Source: CAD feature listing. Evaluate the final solid. Frame: model axes, mm. Face numbers are marked on the shaded views. Coordinates: 2 decimals unless noted, no trailing zeros. Write each loop counter-clockwise with the first axis right and the second up, starting at its lowest first coordinate (ties: lowest second). Pieces come first, ordered by that corner, then holes. Notation, with made-up numbers: M 40.25,72.25 L 80.25,72.25 A31 ccw 80.25,98.25 Z; hole C 52.5,-34.75 d2. An arc over 180 degrees is marked long. Answer as CSV lines item,"result". Start each with the question number.
1. Contact query for a flat-ended pin moving along its axis: pin 1 Ø1 at (y, z) = (5, -1.5) entering from +X. Output: stop coordinate, or through.
2. Section A-A on z = 0. Return the cut outline in (x, y), plus the area to 3 significant figures.
3. Line query: probe 1 along X at (y, z) = (4.25, 0); probe 2 along X at (y, z) = (11, -0.55); probe 3 along Z at (x, y) = (0.7, 11). Output: solid intervals per line, ascending. Write a range as [from, to].
4. Mould query, pull axis Z, two halves, no side actions, for the marked faces 1, 2, 3 and 4. Classes: pulls with the +Z half, pulls with the -Z half, needs draft (parallel to the pull), parting line crosses it, or undercut.
5. Section C-C on x = -0.7. Return the cut outline in (y, z).
6. Section D-D on z = -1.5. Return the cut outline in (x, y), plus the area to 3 significant figures.
Autodesk Inventor part; units mm, degrees
ref_plane "YZ Plane" through (0, 0, 0) normal (1, 0, 0) x (0, 1, 0)
ref_plane "XZ Plane" through (0, 0, 0) normal (0, 1, 0) x (-1, 0, 0)
ref_plane "XY Plane" through (0, 0, 0) normal (0, 0, 1) x (1, 0, 0)
sketch "Sketch1" plane through (0, 0, 0) normal (0, 1, 0) x (-1, 0, 0)
  line L0 (1.5155, -0.875) -> (0, -1.75)
  line L1 (0, -1.75) -> (-1.5155, -0.875)
  line L2 (-1.5155, -0.875) -> (-1.5155, 0.875)
  line L3 (-1.5155, 0.875) -> (0, 1.75)
  line L4 (0, 1.75) -> (1.5155, 0.875)
  line L5 (1.5155, 0.875) -> (1.5155, -0.875)
  point P0 (0, 0)
  point P1 (0, 0)
  dimension "d0" = 1.75
extrude "Extrusion1" add sketch "Sketch1" along normal blind 12
sketch "Sketch2" plane through (0, 12, 0) normal (0, 1, 0) x (1, 0, 0)
  point P0 (0, 0)
  point P1 (0, 0)
hole "Hole1" at (0, 12, 0) direction (0, -1, 0) diameter 2.013 end through all
sketch "Sketch3" plane through (0, 0, 0) normal (0, -1, 0) x (1, 0, 0)
  point P0 (-34.949, 34.34)
  point P1 (0, 0)
  point P2 (-40.6419, -41.3626)
  point P3 (-75.5909, -7.0226)
sketch "Sketch4" plane through (0, 12, 0) normal (0, 1, 0) x (1, 0, 0)
  point P0 (0, 0)
  point P1 (-34.949, -34.34)
  point P2 (-40.6419, 41.3626)
  point P3 (-75.5909, 7.0226)
properties part number "12mm_M2.5_standoff"
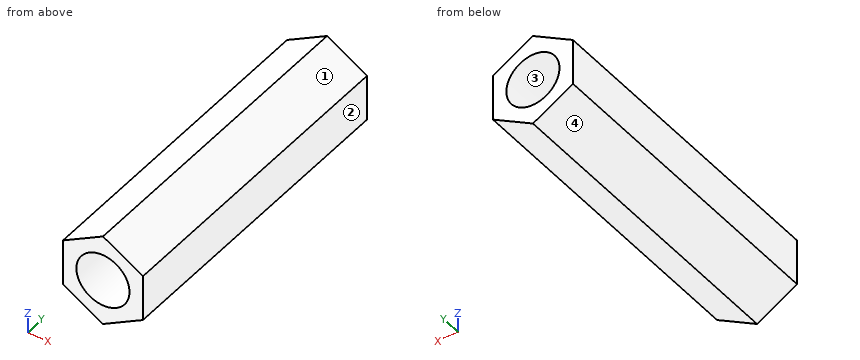
Values:
1,pin 1,"x = 1.3"
2,outline,"M -1.52,0 L -1.01,0 L -1.01,12 L -1.52,12 Z; M 1.01,0 L 1.52,0 L 1.52,12 L 1.01,12 Z"
2,area,"12.2 mm²"
3,probe 1,"[-1.52, -1.01], [1.01, 1.52]"
3,probe 2,"[-1.52, -0.84], [0.84, 1.52]"
3,probe 3,"[-1.35, -0.72], [0.72, 1.35]"
4,face 1,"pulls with the +Z half"
4,face 2,"needs draft"
4,face 3,"undercut"
4,face 4,"pulls with the -Z half"
5,outline,"M 0,-1.35 L 12,-1.35 L 12,-0.72 L 0,-0.72 Z; M 0,0.72 L 12,0.72 L 12,1.35 L 0,1.35 Z"
6,outline,"M -0.43,0 L 0.43,0 L 0.43,12 L -0.43,12 Z"
6,area,"10.4 mm²"
